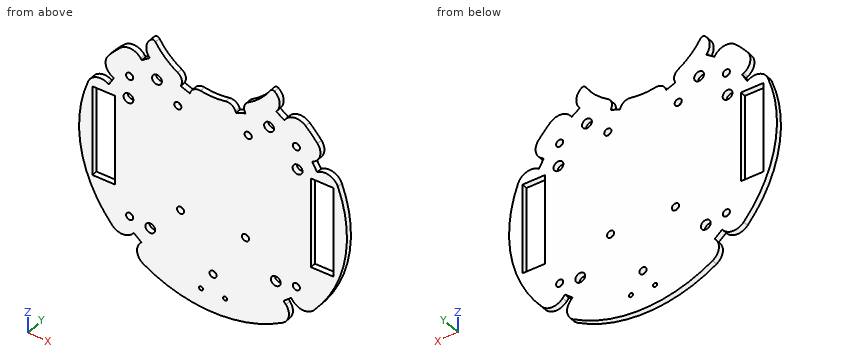
from build123d import *

# Parameters (mm, degrees)
SKETCH1_R           = 2
SKETCH1_R_2         = 1.143
SKETCH1_R_3         = 2.75
SKETCH1_W           = 12.7
SKETCH1_H           = 50.8
BOSS_EXTRUDE1_DEPTH = 3.175


with BuildPart() as part:
    # Sketch1 → Boss-Extrude1 (new body)
    with BuildSketch(Plane(origin=(0, 0, 0), x_dir=(1, 0, 0), z_dir=(0, 1, 0))):
        with BuildLine():
            Line((-36.014757408, -56.228882693), (-35.441180971, -55.409730648))
            Line((-35.441180971, -55.409730648), (-39.946517215, -52.255060249))
            Line((-39.946517215, -52.255060249), (-40.520093651, -53.074212293))
            ThreePointArc((-40.520093651, -53.074212293), (-45.927580176, -56.23617342), (-51.848593315, -54.191543356))
            ThreePointArc((-51.848593315, -54.191543356), (-55.295899374, -50.669157408), (-58.504414423, -46.927960674))
            ThreePointArc((-58.504414423, -46.927960674), (-60.025192689, -40.851285995), (-56.403972981, -35.739974078))
            Line((-56.403972981, -35.739974078), (-55.537947577, -35.239974078))
            Line((-55.537947577, -35.239974078), (-58.287686569, -30.477286437))
            Line((-58.287686569, -30.477286437), (-59.153711973, -30.977286437))
            ThreePointArc((-59.153711973, -30.977286437), (-65.390847794, -31.557698738), (-69.893013303, -27.202328787))
            ThreePointArc((-69.893013303, -27.202328787), (-73.860606951, 13.023468848), (-56.374397975, 49.466425512))
            ThreePointArc((-56.374397975, 49.466425512), (-50.654117331, 52.01932544), (-44.991624855, 49.340690033))
            Line((-44.991624855, 49.340690033), (-44.348837245, 48.57464559))
            Line((-44.348837245, 48.57464559), (-40.135592808, 52.109977443))
            Line((-40.135592808, 52.109977443), (-40.778380417, 52.876021886))
            ThreePointArc((-40.778380417, 52.876021886), (-42.433039833, 58.917628536), (-38.925607882, 64.107698843))
            ThreePointArc((-38.925607882, 64.107698843), (0, 75), (38.925607882, 64.107698843))
            ThreePointArc((38.925607882, 64.107698843), (42.433039833, 58.917628536), (40.778380417, 52.876021886))
            Line((40.778380417, 52.876021886), (39.492805198, 51.343933))
            Line((39.492805198, 51.343933), (43.706049635, 47.808601147))
            Line((43.706049635, 47.808601147), (44.991624855, 49.340690033))
            ThreePointArc((44.991624855, 49.340690033), (50.654117331, 52.01932544), (56.374397975, 49.466425512))
            ThreePointArc((56.374397975, 49.466425512), (73.860606951, 13.023468848), (69.893013303, -27.202328787))
            ThreePointArc((69.893013303, -27.202328787), (65.390847794, -31.557698738), (59.153711973, -30.977286437))
            Line((59.153711973, -30.977286437), (58.287686569, -30.477286437))
            Line((58.287686569, -30.477286437), (55.537947577, -35.239974078))
            Line((55.537947577, -35.239974078), (56.403972981, -35.739974078))
            ThreePointArc((56.403972981, -35.739974078), (60.025192689, -40.851285995), (58.504414423, -46.927960674))
            ThreePointArc((58.504414423, -46.927960674), (55.295899374, -50.669157408), (51.848593315, -54.191543356))
            ThreePointArc((51.848593315, -54.191543356), (45.927580176, -56.23617342), (40.520093651, -53.074212293))
            Line((40.520093651, -53.074212293), (39.946517215, -52.255060249))
            Line((39.946517215, -52.255060249), (35.441180971, -55.409730648))
            Line((35.441180971, -55.409730648), (36.014757408, -56.228882693))
            ThreePointArc((36.014757408, -56.228882693), (37.282182463, -61.682274385), (34.419720881, -66.493943628))
            ThreePointArc((34.419720881, -66.493943628), (33.243515234, -66.777434912), (32.240681933, -66.10056535))
            ThreePointArc((32.240681933, -66.10056535), (26.728650164, -59.250774979), (19.793246149, -53.846860332))
            ThreePointArc((19.793246149, -53.846860332), (17.659799789, -51.192486841), (17.721018114, -47.787557426))
            Line((17.721018114, -47.787557426), (18.078412971, -46.853604046))
            Line((18.078412971, -46.853604046), (12.941669381, -44.887932332))
            Line((12.941669381, -44.887932332), (12.584274523, -45.821885712))
            ThreePointArc((12.584274523, -45.821885712), (10.356790186, -48.397852623), (6.996351286, -48.949887413))
            ThreePointArc((6.996351286, -48.949887413), (0, -48.302004425), (-6.996351286, -48.949887413))
            ThreePointArc((-6.996351286, -48.949887413), (-10.356790186, -48.397852623), (-12.584274523, -45.821885712))
            Line((-12.584274523, -45.821885712), (-12.941669381, -44.887932332))
            Line((-12.941669381, -44.887932332), (-18.078412971, -46.853604046))
            Line((-18.078412971, -46.853604046), (-17.721018114, -47.787557426))
            ThreePointArc((-17.721018114, -47.787557426), (-17.659799789, -51.192486841), (-19.793246149, -53.846860332))
            ThreePointArc((-19.793246149, -53.846860332), (-26.728650164, -59.250774979), (-32.240681933, -66.10056535))
            ThreePointArc((-32.240681933, -66.10056535), (-33.243515234, -66.777434912), (-34.419720881, -66.493943628))
            ThreePointArc((-34.419720881, -66.493943628), (-37.282182463, -61.682274385), (-36.014757408, -56.228882693))
        make_face()
        with Locations((-18.178952795, 24.310551096)):
            Circle(SKETCH1_R, mode=Mode.SUBTRACT)
        with Locations((-46.663733983, -40.081231883)):
            Circle(SKETCH1_R, mode=Mode.SUBTRACT)
        with Locations((46.663733983, -40.081231883)):
            Circle(SKETCH1_R, mode=Mode.SUBTRACT)
        with Locations((46.663733983, 40.081231883)):
            Circle(SKETCH1_R, mode=Mode.SUBTRACT)
        with Locations((-46.663733983, 40.081231883)):
            Circle(SKETCH1_R, mode=Mode.SUBTRACT)
        with Locations((-6.731, 64.107698843)):
            Circle(SKETCH1_R_2, mode=Mode.SUBTRACT)
        with Locations((6.731, 64.107698843)):
            Circle(SKETCH1_R_2, mode=Mode.SUBTRACT)
        with Locations((-31.384508293, -44.821722961)):
            Circle(SKETCH1_R_3, mode=Mode.SUBTRACT)
        with Locations((18.178952795, 24.310551096)):
            Circle(SKETCH1_R, mode=Mode.SUBTRACT)
        with Locations((0, 53.061187965)):
            Circle(SKETCH1_R, mode=Mode.SUBTRACT)
        with Locations((-47.332350097, -27.32734507)):
            Circle(SKETCH1_R_3, mode=Mode.SUBTRACT)
        with Locations((-35.134053633, 41.871134639)):
            Circle(SKETCH1_R_3, mode=Mode.SUBTRACT)
        with Locations((-19.709430746, -34.896815973)):
            Circle(SKETCH1_R, mode=Mode.SUBTRACT)
        with Locations((35.134053633, 41.871134639)):
            Circle(SKETCH1_R_3, mode=Mode.SUBTRACT)
        with Locations((47.332350097, -27.32734507)):
            Circle(SKETCH1_R_3, mode=Mode.SUBTRACT)
        with Locations((31.384508293, -44.821722961)):
            Circle(SKETCH1_R_3, mode=Mode.SUBTRACT)
        with Locations((19.709430746, -34.896815973)):
            Circle(SKETCH1_R, mode=Mode.SUBTRACT)
        with Locations((61.164123727, 0)):
            Rectangle(SKETCH1_W, SKETCH1_H, mode=Mode.SUBTRACT)
        with Locations((-61.164123727, 0)):
            Rectangle(SKETCH1_W, SKETCH1_H, mode=Mode.SUBTRACT)
    extrude(amount=BOSS_EXTRUDE1_DEPTH)


solid = part.part
Input: part model. Units: mm. Frame: model coordinates. Coordinates: 2 decimals unless noted, no trailing zeros. Loops run counter-clockwise (first coordinate to the right, second up) from the corner with the lowest first, then second, coordinate; pieces in that order, holes last. Notation, with made-up numbers: (79, 45) -> (88, 45) arc R26 cw to (88, 74) -> close; hole circle Ø5 at (4, 32.5). An arc over 180 degrees is marked (long way). Write each question's results on one line, items separated by ' | '. Start each with the question number.
Q1. Section C-C, the plane y = 0.6. State how many separate pieces and enclosed holes the cut face has, plus the area to 3 significant figures.
Q2. Ray query, line 1 (Z direction, x = 0, y = 2); line 2 (X direction, y = 2.3, z = 2.5); line 3 (X direction, y = 0.4, z = -8.5). Return the intervals inside material, ascending. Write a range as from..to.
Q3. Section A-A, the plane x = 0. Return the cut outline in (y, z) (3 decimals).
Q4. Section B-B, the plane z = 5. Return the cut outline in (x, y) (3 decimals).
Q5. Pin query (flat end, axial travel): pin 1 (2.5 mm diameter, centred on x = 19.71, z = 34.9, fed in from +Y); pin 2 (7 mm diameter, centred on x = 31.38, z = 44.82, fed in from -Y); pin 3 (1.6 mm diameter, centred on y = 2, z = -9.5, fed in from -X); pin 4 (1.6 mm diameter, centred on x = -62.5, y = 1.5, fed in from +Z). Return the tip coordinate at first contact, or that it passes through.
Found:
1) separate pieces: 1 | enclosed holes: 19 | area: 14,300 mm2
2) line 1: -75..-55.06, -51.06..48.3 | line 2: -74.96..-67.51, -54.81..54.81, 67.51..74.96 | line 3: -74.52..-67.51, -54.81..54.81, 67.51..74.52
3) outline: (0, -75) -> (3.175, -75) -> (3.175, -55.061) -> (0, -55.061) -> close; (0, -51.061) -> (3.175, -51.061) -> (3.175, 48.302) -> (0, 48.302) -> close
4) outline: (-74.833, 0) -> (-67.514, 0) -> (-67.514, 3.175) -> (-74.833, 3.175) -> close; (-54.814, 0) -> (54.814, 0) -> (54.814, 3.175) -> (-54.814, 3.175) -> close; (67.514, 0) -> (74.833, 0) -> (74.833, 3.175) -> (67.514, 3.175) -> close
5) pin 1: through | pin 2: y = 0 | pin 3: x = -74.49 | pin 4: z = 31.98
